```python
from build123d import *

# Parameters (mm, degrees)
F0_W     = 101.6
F0_H     = 38.1
F1_DEPTH = 355.6
F2_W     = 88.9
F2_H     = 19.05
F3_DEPTH = 101.601


with BuildPart() as f1:
    # F0 (on Front) → F1 (new body, symmetric)
    with BuildSketch(Plane.XZ):
        Rectangle(F0_W, F0_H)
    extrude(amount=F1_DEPTH, both=True)

    # F2 (on face) → F3 (cut, through all)
    with BuildSketch(Plane.YZ.offset(50.8)):
        with Locations((311.15, -9.525)):
            Rectangle(F2_W, F2_H)
        with Locations((-311.15, -9.525)):
            Rectangle(F2_W, F2_H)
    extrude(amount=-F3_DEPTH, mode=Mode.SUBTRACT)


solid = f1.part
```
Model file for the job. Use its own axes, mm. A direction names the side the tool comes from. Give positions to 0.01 mm unless a question says otherwise; leave off trailing zeros. Loops run counter-clockwise (first coordinate to the right, second up) from the corner with the lowest first, then second, coordinate; pieces in that order, holes last. Notation, with made-up numbers: (52.5, 64.25) -> (104.5, 64.25) arc R17 cw to (104.5, 85.25) -> close; hole circle Ø3 at (80, 69). An arc over 180 degrees is marked (long way). Use CSV: the item, a comma, the result in double quotes. Start each with the question number.
1) Mould opens along X. For faces 1 (the flat face through (50.8, -5, 0)), 2 (the flat face through (1, 311, 0)), 3 (the flat face through (-50.8, -5, 0)) say: released by +X, released by -X, zero draft, split by the parting line, or undercut.
2) Slice it at A-A on x = -18.5. Give the cut face in (y, z), plus the area to 3 significant figures.
3) Flat gauge pins, fed straight in: pin 1 Ø2 at (x, z) = (-27, -13) entering from -Y; pin 2 Ø2 at (x, z) = (31.5, -11.5) entering from +Y. Where does each tip first touch, or does it go through?
4) Wall check: line 1 (Y direction, x = -41, z = -3); line 2 (Z direction, x = 36.5, y = 311.5). Give the ranges that are in metal, low to high.
5) Tool access for faces 4 (the flat face through (1, 266.7, -10)), 5 (the flat face through (-1, -4, -19.05)), 6 (the flat face through (1, -312, 0)): list every direction of +Z, -Z, +X, -X, +Y, -Y with a clear straight run to the whole face (end or side of a thin tool).
Computed values:
1,face 1,"released by +X"
1,face 2,"zero draft"
1,face 3,"released by -X"
2,outline,"(-355.6, 0) -> (-266.7, 0) -> (-266.7, -19.05) -> (266.7, -19.05) -> (266.7, 0) -> (355.6, 0) -> (355.6, 19.05) -> (-355.6, 19.05) -> close"
2,area,"23,700 mm^2"
3,pin 1,"stops at y = -266.7"
3,pin 2,"stops at y = 266.7"
4,line 1,"y = -266.7 to 266.7"
4,line 2,"z = 0 to 19.05"
5,face 4,"-Z, +X, -X, +Y"
5,face 5,"-Z, +X, -X, +Y, -Y"
5,face 6,"-Z, +X, -X, -Y"
